Design review of the part built by this model. Coordinates are the model's own, in mm. Round coordinates to 2 decimals unless told otherwise and drop trailing zeros. Loops run counter-clockwise (first coordinate to the right, second up) from the corner with the lowest first, then second, coordinate; pieces in that order, holes last. Notation, with made-up numbers: M 31,-26.75 L 79,-26.75 A36 cw 79,9.25 Z; hole C 85,35.25 d4. An arc over 180 degrees is marked long. Use a Markdown table: item, result.
from build123d import *

# Parameters (mm, degrees)
SKETCH2_R          = 6.325
CUT_EXTRUDE1_DEPTH = 35
SKETCH3_R          = 5
CUT_EXTRUDE2_DEPTH = 30
FILLET1_R          = 5


with BuildPart() as part:
    # Sketch1 → Revolve1 (revolve)
    with BuildSketch(Plane.XY):
        with BuildLine():
            Line((0, 0), (0, 60))
            ThreePointArc((0, 60), (30, 30), (0, 0))
        make_face()
    revolve(axis=Axis((0, 0, 0), (0, 1, 0)))

    # Sketch2 → Cut-Extrude1 (cut)
    with BuildSketch(Plane.XY):
        with Locations((0, 30)):
            Circle(SKETCH2_R)
    extrude(amount=-CUT_EXTRUDE1_DEPTH, mode=Mode.SUBTRACT)

    # Sketch3 → Cut-Extrude2 (cut)
    with BuildSketch(Plane(origin=(0, 0, 0), x_dir=(1, 0, 0), z_dir=(0, 1, 0))):
        with Locations(Location((0, 0, 0), (0, 0, 180))):
            Circle(SKETCH3_R)
    extrude(amount=CUT_EXTRUDE2_DEPTH, mode=Mode.SUBTRACT)

    # Fillet1
    # the kernel refuses this fillet: 5 mm, written as the material it takes off along each edge
    with BuildSketch(Plane(origin=(17.5, 30, 0), x_dir=(0, 1, 0), z_dir=(-1, 0, 0))) as fillet1_piece_1_section:
        with BuildLine():
            CenterArc((FILLET1_R, -FILLET1_R), FILLET1_R, 90, 90)
            Line((0, -FILLET1_R), (0, 0))
            Line((0, 0), (FILLET1_R, 0))
        make_face()
    fillet1_piece_1 = extrude(amount=35, mode=Mode.PRIVATE)
    fillet1_piece_1 = fillet1_piece_1 & Plane(origin=(0, 31.17476679, 0), x_dir=(-1, 0, 0), z_dir=(0, -1, 0)) * Cylinder(5, 90, mode=Mode.PRIVATE)
    fillet1_piece_1 = fillet1_piece_1 & Plane(origin=(0, 30, 1.028849853), x_dir=(1, 0, 0), z_dir=(0, 0, 1)) * Cylinder(6.325, 90, mode=Mode.PRIVATE)
    add(fillet1_piece_1, mode=Mode.SUBTRACT)


solid = part.part
1. Take a section at C-C on y = 31.5. Give the boundary of the cut face in (x, z), and give its area (3 significant figures).
Check values:
| item | result |
|---|---|
| outline | M -6.14,-29.33 L -6.14,0 L -5,0 A5 cw -4.79,1.43 L 4.79,1.43 A5 cw 5,0 L 6.14,0 L 6.14,-29.33 A29.96 ccw long Z |
| area | 2,440 mm² |
2. Take a section at A-A on y = 14. Give the boundary of the cut face in (x, z), and give its area (3 significant figures).
Check values:
| item | result |
|---|---|
| outline | C 0,0 d50.75; hole C 0,0 d10 |
| area | 1,940 mm² |
3. Wall thickness on line 1 along Y through (x, z) = (0, -8) (3 decimals); line 2 along Y through (x, z) = (-1, -15.5); line 3 along Z through (x, y) = (0, 8.75): over which ranges is each line inside the solid? List them lowest first. Write a range as from..to.
Check values:
| item | result |
|---|---|
| line 1 | y = 1.086..23.675, 36.325..58.914 |
| line 2 | y = 4.33..23.75, 36.25..55.67 |
| line 3 | z = -21.18..-5, 5..21.18 |
4. Take a section at B-B on z = -11. Give the boundary of the cut face in (x, y) (3 decimals).
Check values:
| item | result |
|---|---|
| outline | C 0,30 d55.821; hole C 0,30 d12.65 |
5. Insertion check: pin 1 (3 mm diameter, centred on y = 23, z = 23, fed in from +X); pin 2 (10 mm diameter, centred on x = -10.5, z = 12.5, fed in from +Y); pin 3 (10 mm diameter, centred on x = -16.5, y = 34.5, fed in from +Z). Each pin has a flat end and moves straight along its axis. Give the tip position at first contact, or say it passes through.
Check values:
| item | result |
|---|---|
| pin 1 | stops at x = 19.8 |
| pin 2 | stops at y = 57.78 |
| pin 3 | stops at z = 27.45 |
6. Take a section at D-D on x = 23. Give the boundary of the cut face in (y, z), and give its area (3 significant figures).
Check values:
| item | result |
|---|---|
| outline | C 30,0 d38.52 |
| area | 1,170 mm² |
